Here's the drawing with two shaded views (mm, measured from the low corner). I have some questions. A direction names the side the tool comes from. Round coordinates to 2 decimals unless told otherwise and drop trailing zeros. Write each loop counter-clockwise with the first axis right and the second up, starting at its lowest first coordinate (ties: lowest second). Pieces come first, ordered by that corner, then holes. Notation, with made-up numbers: (-6, -18.5) - (5, -18.5) arc R22 cw to (5, 20.5) - close; hole circle Ø4 at (55, 12). An arc over 180 degrees is marked (long way). Return JSON: item names as keys, results as strings. Group by question number.
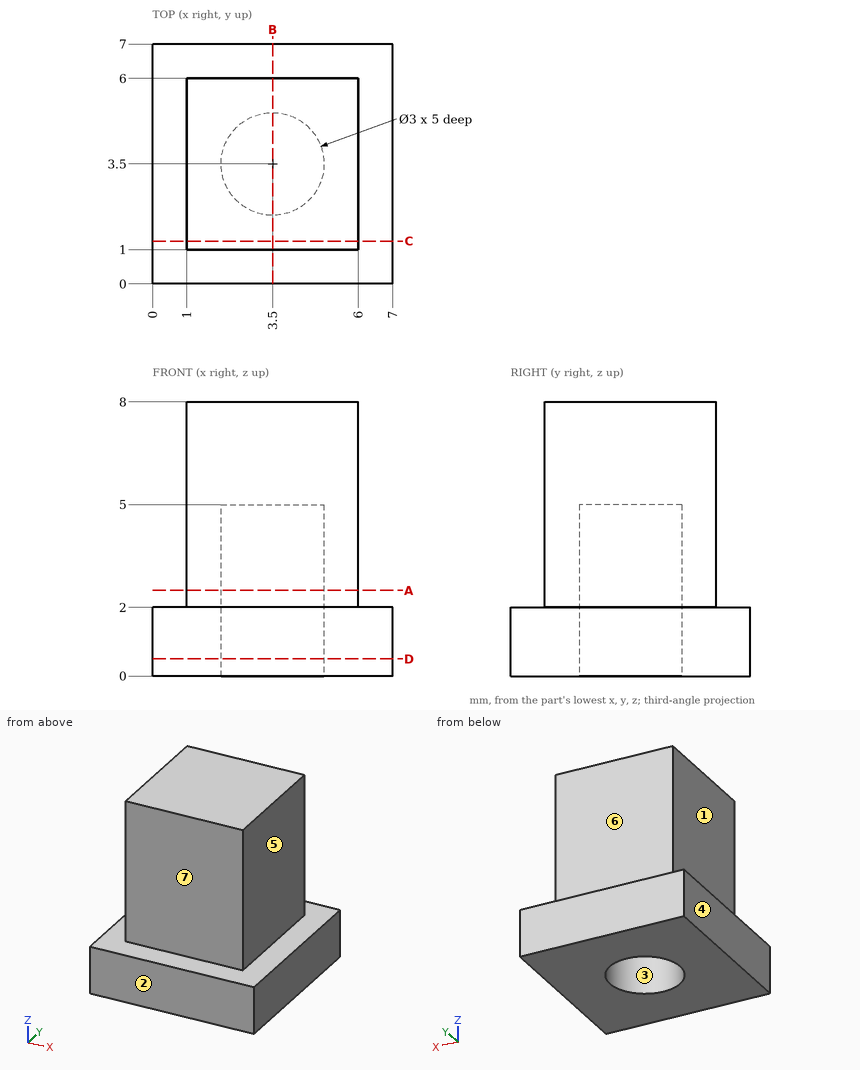
1) Imagine slicing it at A-A (z = 2.5). Please give me the cut outline in (x, y), plus the area to 3 significant figures.
2) Imagine slicing it at D-D (z = 0.5). Please give me the cut outline in (x, y).
3) Imagine slicing it at B-B (x = 3.5). Please give me the cut outline in (y, z), plus the area to 3 significant figures.
4) If we mould it in two halves opening along Y, with no side actions, what happens to the marked faces 1, 2 and 3? For each: released by +Y, released by -Y, zero draft, split by the parting line, or undercut.
5) Imagine slicing it at C-C (y = 1.25). Please give me the cut outline in (x, z).
6) For the marked faces 4, 5, 6 and 7, which set-ups out of +Z, -Z, +X, -X, +Y, -Y let a thin tool reach every point of the face, with its end or its side?
7) Will these pins go through, and if not, where does the flat tip stop? pin 1 Ø3 at (x, y) = (6, 3.5) entering from -Z; pin 2 Ø4 at (x, z) = (4, 5.5) entering from -Y; pin 3 Ø2.5 at (y, z) = (2.5, 4.5) entering from +X; pin 4 Ø1.5 at (x, z) = (2, 5.5) entering from +Y.
8) I need wall thicknesses on line 1 along Y through (x, z) = (3.5, 3.95); line 2 along X through (y, z) = (2.75, 6.75); line 3 along Z through (x, y) = (3, 4). Which ranges of each line are inside material? Lowest first, please.
Results found:
{
 "1": {"outline": "(1, 1) - (6, 1) - (6, 6) - (1, 6) - close; hole circle Ø3 at (3.5, 3.5)", "area": "17.9 mm²"},
 "2": {"outline": "(0, 0) - (7, 0) - (7, 7) - (0, 7) - close; hole circle Ø3 at (3.5, 3.5)"},
 "3": {"outline": "(0, 0) - (2, 0) - (2, 5) - (5, 5) - (5, 0) - (7, 0) - (7, 2) - (6, 2) - (6, 8) - (1, 8) - (1, 2) - (0, 2) - close", "area": "29.0 mm²"},
 "4": {"face 1": "zero draft", "face 2": "released by -Y", "face 3": "undercut"},
 "5": {"outline": "(0, 0) - (7, 0) - (7, 2) - (6, 2) - (6, 8) - (1, 8) - (1, 2) - (0, 2) - close"},
 "6": {"face 4": "+Z, -Z, -X, +Y, -Y", "face 5": "+Z, +X, +Y, -Y", "face 6": "+Z, +X, -X, +Y", "face 7": "+Z, +X, -X, -Y"},
 "7": {"pin 1": "stops at z = 0", "pin 2": "stops at y = 1", "pin 3": "stops at x = 6", "pin 4": "stops at y = 6"},
 "8": {"line 1": "y = 1 to 2, 5 to 6", "line 2": "x = 1 to 6", "line 3": "z = 5 to 8"}
}
